Design review of the part built by this model. Coordinates are the model's own, in mm. Give positions to 0.01 mm unless a question says otherwise; leave off trailing zeros. Order: outer loops, then holes, each group sorted by start corner. A loop starts at its lowest first (then second) coordinate and runs counter-clockwise, first axis right, second up. Notation, with made-up numbers: M 84,-24 L 140,-24 A11 ccw 140,-10 Z; hole C -15,7 d9. An arc over 180 degrees is marked long. Put each result on its own line as item: value. Start each with the question number.
from build123d import *

# Parameters (mm, degrees)
F1_W     = 71.663826704
F1_H     = 64.8628622293
F2_DEPTH = 73.2403695583
F5_R     = 12.1768440653


# Not quite as in the source:
# - the program builds the solid bodies; features that only make, move or delete a surface that nothing else refers to are left out


with BuildPart() as f2:
    # F1 (on face) → F2 (new body)
    with BuildSketch(Plane.XZ):
        with Locations((1.3996511698, -0.3036260605)):
            Rectangle(F1_W, F1_H)
    extrude(amount=F2_DEPTH)

    # F5
    f5_edges = [f2.edges().sort_by_distance(p)[0] for p in [
        (-34.432262, -36.620185, -32.735057),
        (37.231565, -36.620185, -32.735057),
        (-34.432262, -36.620185, 32.127805),
        (-34.432262, -73.24037, -0.303626),
        (1.399651, -73.24037, 32.127805),
        (37.231565, -73.24037, -0.303626),
        (1.399651, -73.24037, -32.735057),
    ]]
    fillet(f5_edges, radius=F5_R)


solid = f2.part
1. Consider section B-B on x = -26.5. Give the boundary of the cut face in (y, z).
2. Consider section D-D on y = -64. Give the boundary of the cut face in (x, z).
3. Insertion check: pin 1 (1.5 mm diameter, centred on x = 13, z = -24, fed in from -Y); pin 2 (2 mm diameter, centred on x = -24.5, y = -27, fed in from +Z). Each pin has a flat end and moves straight along its axis. Give the tip position at first contact, or say it passes through.
4. Consider section A-A on y = -18. Give the boundary of the cut face in (x, z), then the cut area to 3 significant figures.
5. The part is to be moulded in two halves that separate along Z. For faces 1 (the cylindrical face through (33.76, -69.58, 6.15)), 2 (the cylindrical face through (33.57, -30.96, -29.26)), 3 (the cylindrical face through (7.904, -69.579, 28.655)), say which applies: +Z half, -Z half, draft (parallel to the pull), parting line (faces both ways), or undercut.
6. Consider section C-C on z = 22. Give the boundary of the cut face in (x, y), then the cut area to 3 significant figures.
7. To check wall thickness, follow probe 1 along Y at (x, z) = (-27.5, -16); probe 2 along Y at (x, z) = (33, -10); probe 3 along Z at (x, y) = (-29, -53.5). State the ranges of each line that lie inside material, in increasing order.
Returned:
1. outline: M -72.48,-20.56 A11.41 ccw -61.06,-31.97 L 0,-31.97 L 0,31.36 L -61.06,31.36 A11.41 ccw -72.48,19.95 Z
2. outline: M -34.07,-20.56 A11.82 ccw -22.26,-32.38 L 25.05,-32.38 A11.82 ccw 36.87,-20.56 L 36.87,31.77 L -22.26,31.77 A11.82 ccw -34.07,19.95 Z
3. pin 1: stops at y = -72.94
3. pin 2: stops at z = 32.06
4. outline: M -34.43,-20.56 A12.18 ccw -22.26,-32.74 L 25.05,-32.74 A12.18 ccw 37.23,-20.56 L 37.23,32.13 L -22.26,32.13 A12.18 ccw -34.43,19.95 Z
4. area: 4,550 mm2
5. face 1: draft
5. face 2: -Z half
5. face 3: +Z half
6. outline: M -34.26,-61.06 A12 ccw -22.26,-73.07 L 27.1,-73.07 A12.18 ccw 37.23,-61.06 L 37.23,0 L -34.26,0 Z
6. area: 5,160 mm2
7. probe 1: y = -72.05 to 0
7. probe 2: y = -70.29 to 0
7. probe 3: z = -30.7 to 30.09
